Design review of the part built by this model. Coordinates are the model's own, in mm. Face numbers are marked on the shaded views. A direction names the side the tool comes from. Round coordinates to 2 decimals unless told otherwise and drop trailing zeros. Order: outer loops, then holes, each group sorted by start corner. A loop starts at its lowest first (then second) coordinate and runs counter-clockwise, first axis right, second up. Notation, with made-up numbers: M -17,-25 L 5,-25 A15 ccw 5,-17 Z; hole C 65.25,77.5 d11. An arc over 180 degrees is marked long. Write each question's results on one line, items separated by ' | '. Start each with the question number.
Item 1: Take a section at C-C, the plane x = 29.5. Write out the cut boundary in (y, z).
Item 2: The part is to be moulded in two halves that separate along X. For the marked faces 4, 5 and 6, say which applies: +X half, -X half, draft (parallel to the pull), parting line (faces both ways), or undercut.
Item 3: Take a section at A-A, the plane z = 8.25. Write out the cut boundary in (x, y).
Item 4: Machinability: for the marked faces 1, 2 and 3, which of the approach directions +Z, -Z, +X, -X, +Y, -Y give a long, thin tool a straight path to every point of the face, cutting with its end or side? Answer none if there is none.
Item 5: Wall thickness on line 1 (Y direction, x = 30.5, z = 8.5); line 2 (Y direction, x = 6, z = 13.5); line 3 (Y direction, x = 25, z = 1.5): over which ranges is each line inside the solid? List them lowest first. Write a range as [from, to].
Item 6: Take a section at B-B, the plane y = -30.5. Write out the cut boundary in (x, z).
Item 7: Take a section at D-D, the plane y = -23.5. Write out the cut boundary in (x, z).
Item 8: Clearance check with flat-ended pins moving along their axes: pin 1 (4 mm diameter, centred on x = 30.5, y = -32, fed in from +Z); pin 2 (4.5 mm diameter, centred on x = 19, y = -18.5, fed in from -Z); pin 3 (9.5 mm diameter, centred on x = 8.5, y = -32.5, fed in from +Z); pin 4 (4.5 mm diameter, centred on x = 7.5, y = -10.5, fed in from +Z). State where each tip first meets the part, or that it passes through.
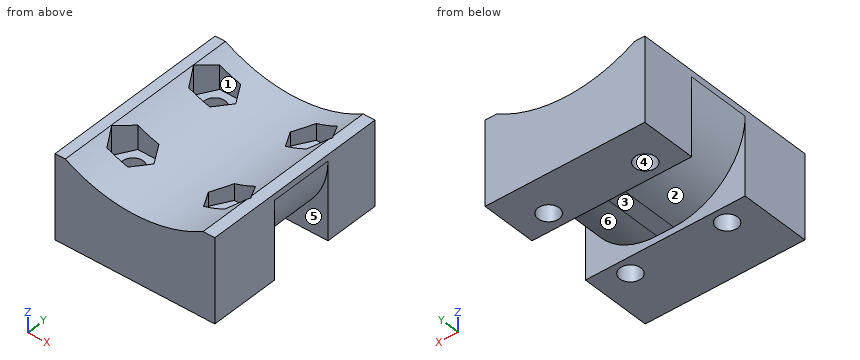
```python
from build123d import *

# Parameters (mm, degrees)
F0_W      = 38
F0_H      = 45
F1_DEPTH  = 20
F0_R      = 2.5
F2_DEPTH  = 13
F3_DEPTH  = 13
F4_DEPTH  = 13
F5_DEPTH  = 13
F6_W      = 15
F6_H      = 20
F7_DEPTH  = 40.2
F9_R      = 32.5
F10_DEPTH = 102.8
F11_R     = 17


with BuildPart() as f1:
    # F0 (on Top) → F1 (new body)
    with BuildSketch(Plane.XY):
        with Locations((19, -22.5)):
            Rectangle(F0_W, F0_H)
        Polygon((12.5229473419, -32), (10.011473671, -36.35), (4.988526329, -36.35), (2.4770526581, -32), (4.988526329, -27.65), (10.011473671, -27.65), align=None, mode=Mode.SUBTRACT)
        Polygon((35.5229473419, -32), (33.011473671, -36.35), (27.988526329, -36.35), (25.4770526581, -32), (27.988526329, -27.65), (33.011473671, -27.65), align=None, mode=Mode.SUBTRACT)
        Polygon((2.4770526581, -9), (4.988526329, -4.65), (10.011473671, -4.65), (12.5229473419, -9), (10.011473671, -13.35), (4.988526329, -13.35), align=None, mode=Mode.SUBTRACT)
        Polygon((25.4770526581, -9), (27.988526329, -4.65), (33.011473671, -4.65), (35.5229473419, -9), (33.011473671, -13.35), (27.988526329, -13.35), align=None, mode=Mode.SUBTRACT)
    extrude(amount=F1_DEPTH)

    # F0 (on Top) → F2 (join)
    with BuildSketch(Plane.XY):
        Polygon((10.011473671, -4.65), (4.988526329, -4.65), (2.4770526581, -9), (4.988526329, -13.35), (10.011473671, -13.35), (12.5229473419, -9), align=None)
        with Locations((7.5, -9)):
            Circle(F0_R, mode=Mode.SUBTRACT)
    extrude(amount=F2_DEPTH)

    # F0 (on Top) → F3 (join)
    with BuildSketch(Plane.XY):
        Polygon((33.011473671, -4.65), (27.988526329, -4.65), (25.4770526581, -9), (27.988526329, -13.35), (33.011473671, -13.35), (35.5229473419, -9), align=None)
        with Locations((30.5, -9)):
            Circle(F0_R, mode=Mode.SUBTRACT)
    extrude(amount=F3_DEPTH)

    # F0 (on Top) → F4 (join)
    with BuildSketch(Plane.XY):
        Polygon((4.988526329, -36.35), (10.011473671, -36.35), (12.5229473419, -32), (10.011473671, -27.65), (4.988526329, -27.65), (2.4770526581, -32), align=None)
        with Locations((7.5, -32)):
            Circle(F0_R, mode=Mode.SUBTRACT)
    extrude(amount=F4_DEPTH)

    # F0 (on Top) → F5 (join)
    with BuildSketch(Plane.XY):
        Polygon((27.988526329, -36.35), (33.011473671, -36.35), (35.5229473419, -32), (33.011473671, -27.65), (27.988526329, -27.65), (25.4770526581, -32), align=None)
        with Locations((30.5, -32)):
            Circle(F0_R, mode=Mode.SUBTRACT)
    extrude(amount=F5_DEPTH)

    # F6 (on Right) → F7 (cut)
    with BuildSketch(Plane.YZ):
        with Locations((-20.6906894967, -8.5)):
            Rectangle(F6_W, F6_H)
    extrude(amount=F7_DEPTH, mode=Mode.SUBTRACT)

    # F9 (on offset) → F10 (cut)
    with BuildSketch(Plane.XZ.offset(70)):
        with Locations((18.8195854425, 48.0670109391)):
            Circle(F9_R)
    extrude(amount=-F10_DEPTH, mode=Mode.SUBTRACT)

    # F11
    f11_edges = [f1.edges().sort_by_distance(p)[0] for p in [
        (38, -20.690689, 1.5),
        (0, -20.690689, 1.5),
    ]]
    fillet(f11_edges, radius=F11_R)


solid = f1.part
```
Results list:
1) outline: M -45,0 L -34.29,0 L -34.29,13 L -36.35,13 L -36.35,17.37 L -45,17.37 Z; M -29.71,0 L -28.19,0 L -28.19,3.78 L -13.19,3.78 L -13.19,0 L -11.29,0 L -11.29,13 L -13.35,13 L -13.35,17.37 L -27.65,17.37 L -27.65,13 L -29.71,13 Z; M -6.71,0 L 0,0 L 0,17.37 L -4.65,17.37 L -4.65,13 L -6.71,13 Z
2) face 4: undercut | face 5: draft | face 6: +X half
3) outline: M 0,-45 L 38,-45 L 38,-28.19 L 34.56,-28.19 L 34.56,-13.19 L 38,-13.19 L 38,0 L 0,0 L 0,-13.19 L 3.44,-13.19 L 3.44,-28.19 L 0,-28.19 Z; hole C 7.5,-32 d5; hole C 7.5,-9 d5; hole C 30.5,-32 d5; hole C 30.5,-9 d5
4) face 1: +Z | face 2: -Z, -X | face 3: -Z, +X, -X
5) line 1: [-45, -34.5], [-29.5, -11.5], [-6.5, 0] | line 2: [-45, -36.35], [-27.65, -13.35], [-4.65, 0] | line 3: [-45, -28.19], [-13.19, 0]
6) outline: M 0,0 L 5.5,0 L 5.5,13 L 3.34,13 L 3.34,19.49 A32.5 cw 2.43,20 L 0,20 Z; M 9.5,0 L 28.5,0 L 28.5,13 L 26.34,13 L 26.34,16.45 A32.5 cw 11.66,16.37 L 11.66,13 L 9.5,13 Z; M 32.5,0 L 38,0 L 38,20 L 35.21,20 A32.5 cw 34.66,19.69 L 34.66,13 L 32.5,13 Z
7) outline: M 0,18.5 A17 ccw 17,1.5 L 21,1.5 A17 ccw 38,18.5 L 38,20 L 35.21,20 A32.5 cw 2.43,20 L 0,20 Z
8) pin 1: through | pin 2: z = 1.5 | pin 3: z = 18.32 | pin 4: z = 13
